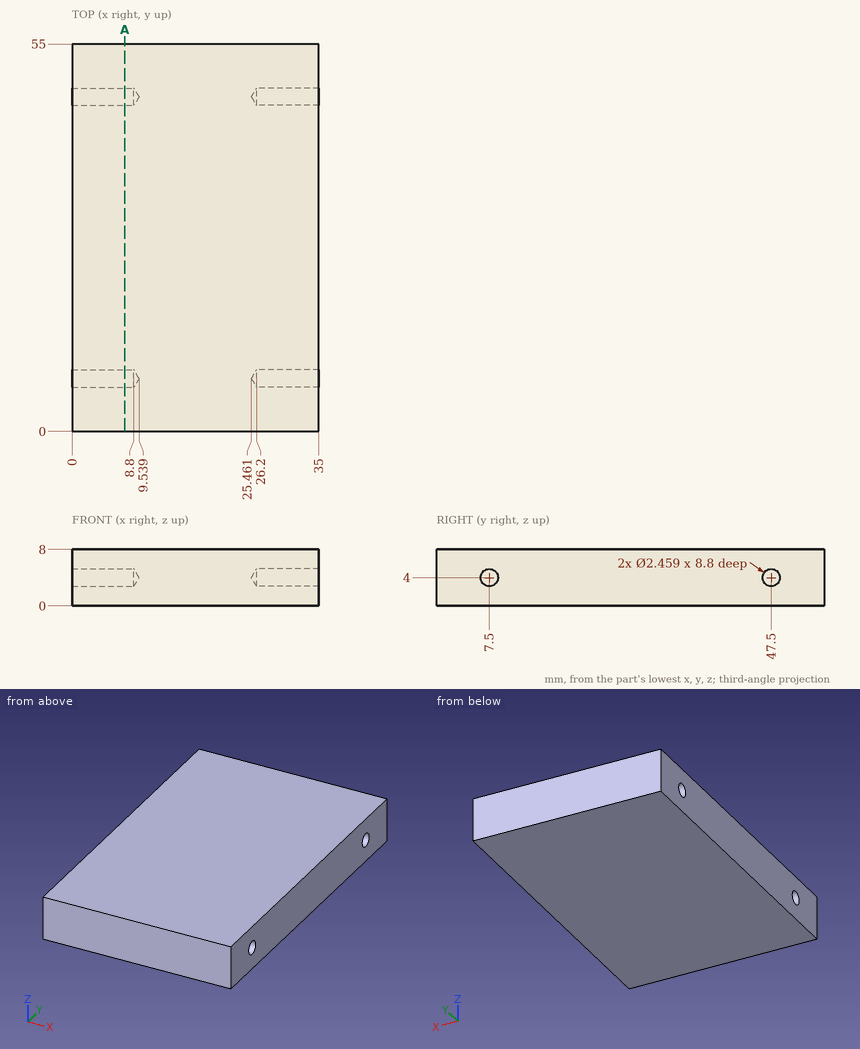
Study the drawing (mm; zero at the part's minimum x, y, z) and answer. Coordinates: 2 decimals unless noted, no trailing zeros. Order: outer loops, then holes, each group sorted by start corner. A loop starts at its lowest first (then second) coordinate and runs counter-clockwise, first axis right, second up. Notation, with made-up numbers: M -38.5,66 L -3.5,66 A34 cw -3.5,98 Z; hole C 9,37.5 d8. An arc over 180 degrees is marked long. Answer as a JSON object with one key per item and string values. Group by question number.
1. Section A-A on x = 7.5 is taken. Write down the section's boundary in (y, z).
2. Straight lines are drawn through the part: line 1 (Y direction, x = 33, z = 4); line 2 (Z direction, x = 6, y = 47.5); line 3 (Z direction, x = 33, y = 47). For each, find the intervals that lie inside material, in ascending order.
3. Flat-ended cylindrical pins translate along their axes: P1, Ø1.5, axis at y = 7.5, z = 4, coming from the +X side; P2, Ø2, axis at y = 47.5, z = 4, coming from the +X side; P3, Ø2, axis at y = 7.5, z = 4, coming from the -X side. Find the tip coordinate at first contact, or state that the pin passes through.
Values follow:
{
 "1": {"outline": "M 0,0 L 55,0 L 55,8 L 0,8 Z; hole C 7.5,4 d2.46; hole C 47.5,4 d2.46"},
 "2": {"line 1": "0 to 6.27, 8.73 to 46.27, 48.73 to 55", "line 2": "0 to 2.77, 5.23 to 8", "line 3": "0 to 2.88, 5.12 to 8"},
 "3": {"P1": "x = 25.91", "P2": "x = 26.06", "P3": "x = 8.94"}
}
